The listing builds one solid part. Answer for the finished solid, in the listing's coordinates (mm). A direction names the side the tool comes from. Give positions to 0.01 mm unless a question says otherwise; leave off trailing zeros. Order: outer loops, then holes, each group sorted by start corner. A loop starts at its lowest first (then second) coordinate and runs counter-clockwise, first axis right, second up. Notation, with made-up numbers: M 4.25,-29.75 L 26.25,-29.75 A35 cw 26.25,7.25 Z; hole C 47.25,39.5 d3. An arc over 180 degrees is marked long. Answer as a JSON object with one key per item and string values. Group by question number.
```python
from build123d import *

# Parameters (mm, degrees)
CUT_EXTRUDE1_DEPTH = 10
SCALE1_SCALE       = 0.5


with BuildPart() as part:
    # Sketch1 → Revolve1 (revolve)
    with BuildSketch(Plane.XY):
        Polygon((7.5, 0), (7.5, 8), (13.5, 8), (13.5, 6), (9.5, 6), (9.5, 0), align=None)
    revolve(axis=Axis((0, 0, 0), (0, 1, 0)))

    # Sketch2 → Cut-Extrude1 (cut)
    with BuildSketch(Plane(origin=(0, 0, 0), x_dir=(1, 0, 0), z_dir=(0, 1, 0))):
        Polygon((-9.091166867, -15.746362913), (0, 0), (8.625529774, -14.939855811), align=None)
    extrude(amount=CUT_EXTRUDE1_DEPTH, mode=Mode.SUBTRACT)


with BuildPart() as part_1:
    # Scale1: scaled about (0, 0, 0)
    add(part.part.scale(SCALE1_SCALE))


solid = part_1.part
```
Item 1: Section C-C (z = 3.5) is taken. Determine the outline of the cut face in (x, y), and give its area (3 significant figures).
Item 2: A tool of negligible diameter and unlimited length cuts with its end or side. For faces 5 (the cylindrical face through (0.174, 1.479, -4.747)), 6 (the flat face through (2.28, 2.42, 3.95)), 7 (the flat face through (-1, 0, -4)), from which of +Z, -Z, +X, -X, +Y, -Y can it reach the whole face along a straight path? Write none if from no direction.
Item 3: A flat-ended cylindrical pin translates along its axis: P1, Ø1, axis at x = 1.5, z = 0, coming from the +Y side. Find the tip coordinate at first contact, or state that the pin passes through.
Item 4: Section A-A (z = 0) is taken. Determine the outline of the cut face in (x, y), and give its area (3 significant figures).
Item 5: Section D-D (y = 3.4) is taken. Determine the outline of the cut face in (x, z) (3 decimals).
Item 6: Consider probe 1 along Y at (x, z) = (6, 0.5); probe 2 along Z at (x, y) = (0, 1.05); probe 3 along X at (y, z) = (3.15, 3.5). Determine where each line is inside the solid, lowest interval first. Write a range as from..to.
Item 7: Determine the mould class of faces 1 (the flat face through (-2.136, 2.416, 3.699)), 2 (the flat face through (0, 4, -5)), 3 (the cylindrical face through (0.137, 2.028, -3.747)), 4 (the cylindrical face through (0.247, 3.493, -6.745)) for opening direction Z: released by +Z, released by -Z, zero draft, split by the parting line, or undercut.
Item 8: Section B-B (x = 0) is taken. Determine the outline of the cut face in (y, z), and give its area (3 significant figures).
Values found:
{
 "1": {"outline": "M -5.77,3 L -3.21,3 L -3.21,0 L -2.02,0 L -2.02,4 L -5.77,4 Z; M 2.02,0 L 3.21,0 L 3.21,3 L 5.77,3 L 5.77,4 L 2.02,4 Z", "area": "14.6 mm^2"},
 "2": {"face 5": "-Y", "face 6": "+Z, +Y, -Y", "face 7": "+Z, -Z, +X, -X, -Y"},
 "3": {"P1": "passes through"},
 "4": {"outline": "M -6.75,3 L -4.75,3 L -4.75,0 L -3.75,0 L -3.75,4 L -6.75,4 Z; M 3.75,0 L 4.75,0 L 4.75,3 L 6.75,3 L 6.75,4 L 3.75,4 Z", "area": "12.0 mm^2"},
 "5": {"outline": "M -3.375,5.846 A6.75 ccw long 3.375,5.846 L 1.875,3.248 A3.75 cw long -1.875,3.248 Z"},
 "6": {"probe 1": "y = 3..4", "probe 2": "z = -4.75..-3.75", "probe 3": "x = -5.77..-2.02, 2.02..5.77"},
 "7": {"face 1": "released by +Z", "face 2": "zero draft", "face 3": "undercut", "face 4": "split by the parting line"},
 "8": {"outline": "M 0,-4.75 L 3,-4.75 L 3,-6.75 L 4,-6.75 L 4,-3.75 L 0,-3.75 Z", "area": "6.00 mm^2"}
}
